Source: CAD feature listing. Evaluate the final solid. Frame: model axes, mm. A direction names the side the tool comes from. Round coordinates to 2 decimals unless told otherwise and drop trailing zeros. Loops run counter-clockwise (first coordinate to the right, second up) from the corner with the lowest first, then second, coordinate; pieces in that order, holes last. Notation, with made-up numbers: (69, 8) -> (108, 8) arc R11 cw to (108, 26) -> close; hole circle Ø11 at (60, -20). An arc over 180 degrees is marked (long way). Write item = value, one per line.
Autodesk Inventor part; units mm, degrees
ref_plane "YZ Plane" through (0, 0, 0) normal (1, 0, 0) x (0, 1, 0)
ref_plane "XZ Plane" through (0, 0, 0) normal (0, 1, 0) x (-1, 0, 0)
ref_plane "XY Plane" through (0, 0, 0) normal (0, 0, 1) x (1, 0, 0)
sketch "Base" plane through (0, 0, 0) normal (0, 0, 1) x (1, 0, 0)
  circle A0 centre (0, 0) radius 2
  line L0 (-4.5, 5) -> (4.5, 5)
  line L1 (4.5, 5) -> (4.5, -5)
  line L2 (4.5, -5) -> (-4.5, -5)
  line L3 (-4.5, -5) -> (-4.5, 5)
  line L4 (4.5, 0) -> (-4.5, 0) construction
  line L5 (4.5, 10) -> (41.5, 10)
  line L6 (41.5, 10) -> (41.5, -10)
  line L7 (41.5, -10) -> (4.5, -10)
  line L8 (4.5, -10) -> (4.5, 10)
  dimension "d0" = 4
  dimension "d1" = 10
  dimension "d2" = 9
  dimension "d3" = 20
  dimension "d4" = 37
extrude "Extrusion1" add sketch "Base" along normal mid plane 8 contours L0 L1 L2 L3
extrude "Extrusion2" add sketch "Base" along normal mid plane 15 contours L8 L5 L6 L7 L1
fillet "Fillet1" radius 4 2 edges at (-4.5, -5, 0) (-4.5, 5, 0)
fillet "Fillet2" radius 1 2 edges at (4.5, 10, 0) (4.5, -10, 0)
sketch "Sketch2" plane through (0, 0, 7.5) normal (0, 0, 1) x (1, 0, 0)
  arc A0 (4.5, -9) -> (5.5, -10) centre (5.5, -9) ccw
  line L0 (5.5, -10) -> (41.5, -10)
  line L1 (41.5, -10) -> (41.5, 10)
  line L2 (41.5, 10) -> (5.5, 10)
  arc A1 (5.5, 10) -> (4.5, 9) centre (5.5, 9) ccw
  line L3 (4.5, 9) -> (4.5, -9)
  line L4 (32.7998, 10) -> (33.5, 9)
  line L5 (33.5, 9) -> (41.5, 9)
  line L6 (41.5, -10) -> (41.5, 10)
  line L7 (41.5, 10) -> (5.5, 10)
  point P0 (0, 0)
  dimension "d11" = 1
  dimension "d12" = 8
  dimension "d13" = 125
extrude "Extrusion3" cut sketch "Sketch2" against normal up to surface (15 mm away) contours L5 L4 L2 L1
fillet "Fillet3" radius 0.5 2 edges at (32.7998, 10, 0) (33.5, 9, 0)
sketch "Sketch3" plane through (41.5, -10, 7.5) normal (1, 0, 0) x (0, 0, -1)
  line L0 (15, 19) -> (0, 19) construction
  line L1 (7.5, 19) -> (7.5, 0) construction
  line L2 (0, 0) -> (15, 0) construction
  line L3 (1.625, 14.625) -> (13.375, 14.625) construction
  line L4 (13.375, 14.625) -> (13.375, 4.375)
  line L5 (13.375, 4.375) -> (1.625, 4.375) construction
  line L6 (1.625, 4.375) -> (1.625, 14.625)
  line L7 (0, 0) -> (0, 19) construction
  line L8 (0, 9.5) -> (15, 9.5) construction
  line L9 (15, 19) -> (15, 0) construction
  arc A0 (13.375, 14.625) -> (1.625, 14.625) centre (7.5, 10.3724) ccw
  arc A1 (1.625, 4.375) -> (13.375, 4.375) centre (7.5, 8.6276) ccw
  point P0 (7.5, 10)
  point P1 (7.5, 14.625)
  point P2 (1.625, 9.5)
  point P3 (7.5, 17.625)
  point P4 (7.5, 1.375)
  dimension "d17" = 11.75
  dimension "d18" = 3
  dimension "d21" = 16.25
extrude "Extrusion4" add sketch "Sketch3" along normal blind 56.5
sketch "Sketch4" plane through (98, -10, 7.5) normal (1, 0, 0) x (0, 0, -1)
  line L0 (13.375, 4.375) -> (13.375, 14.625)
  arc A0 (13.375, 14.625) -> (1.625, 14.625) centre (7.5, 10.3724) ccw
  line L1 (1.625, 14.625) -> (1.625, 4.375)
  arc A1 (1.625, 4.375) -> (13.375, 4.375) centre (7.5, 8.6276) ccw
  arc A2 (12.875, 14.4598) -> (2.125, 14.4598) centre (7.5, 10.3724) ccw
  line L2 (12.875, 14.4598) -> (12.875, 4.5402)
  arc A3 (2.125, 4.5402) -> (12.875, 4.5402) centre (7.5, 8.6276) ccw
  line L3 (2.125, 4.5402) -> (2.125, 14.4598)
  point P0 (7.5, 10)
  dimension "d22" = 0.5
extrude "Extrusion5" add sketch "Sketch4" along normal blind 0.25 contours L2 A3 L3 A2
sketch "Sketch5" plane through (98.25, -10, 7.5) normal (1, 0, 0) x (0, 0, -1)
  arc A0 (13.375, 14.625) -> (1.625, 14.625) centre (7.5, 10.3724) ccw
  line L0 (1.625, 14.625) -> (1.625, 4.375)
  arc A1 (1.625, 4.375) -> (13.375, 4.375) centre (7.5, 8.6276) ccw
  line L1 (13.375, 4.375) -> (13.375, 14.625)
  point P0 (7.5, 10)
extrude "Extrusion6" add sketch "Sketch5" along normal blind 1.75
sketch "Sketch6" plane through (100, -10, 7.5) normal (1, 0, 0) x (0, 0, -1)
  circle A0 centre (7.5, 10) radius 4.5
  dimension "d27" = 9
extrude "Extrusion7" cut sketch "Sketch6" against normal blind 50
sketch "Sketch7" plane through (41.5, -5.625, 5.875) normal (0, 0, 1) x (1, 0, 0)
  line L0 (58.5, 0) -> (58.5, 10.25)
  line L1 (58.5, 5.125) -> (54.5, 5.125) construction
  circle A0 centre (52.5, 5.125) radius 2
  line L2 (52.5, 5.125) -> (54.5, 5.125) construction
  point P0 (-41.5, 5.625)
  dimension "d31" = 4
  dimension "d30" = 4
extrude "Extrusion8" cut sketch "Sketch7" against normal through all
properties part number "LA-T8-1215-50 105-64 Body"
1. Section query B-B (x = 78). Return the cut outline in (y, z) (3 decimals), then the cut area to 3 significant figures.
Evaluation:
outline = (-5.625, -5.875) -> (4.625, -5.875) arc R7.253 ccw to (4.625, 5.875) -> (-5.625, 5.875) arc R7.253 ccw to start; hole circle Ø9 at (0, 0)
area = 106 mm²
2. Set-up query: faces 1 (the face through (2, 1, -4)), 2 (the face through (2, -5, 0)), 3 (the face through (69.354, -8.624, -0.096)). Return all of +Z, -Z, +X, -X, +Y, -Y with unobstructed straight access to the full face (end or side cutting, diameter ignored); none if empty.
Evaluation:
face_1 = -Z, -X, +Y, -Y
face_2 = +Z, -Z, -X, -Y
face_3 = +X, -Y
3. Section query C-C (x = 94). Return the cut outline in (y, z) (3 decimals).
Evaluation:
outline = (-5.625, -5.875) -> (-2.5, -5.875) -> (-2.5, -3.742) arc R4.5 cw to (-2.5, 3.742) -> (-2.5, 5.875) -> (-5.625, 5.875) arc R7.253 ccw to start; (1.5, -5.875) -> (4.625, -5.875) arc R7.253 ccw to (4.625, 5.875) -> (1.5, 5.875) -> (1.5, 4.243) arc R4.5 cw to (1.5, -4.243) -> close
4. Mould query, pull axis X, two halves, no side actions, for faces 4 (the face through (94.923, -2.274, 5.06)), 5 (the face through (50, 0, 0)), 6 (the face through (2, 1, 4)). Classes: released by +X, released by -X, zero draft, split by the parting line, or undercut.
Evaluation:
face_4 = undercut
face_5 = released by +X
face_6 = zero draft
5. Line query: probe 1 along X at (y, z) = (-0.5, 5.25); probe 2 along Y at (x, z) = (0, 0.75); probe 3 along Z at (x, y) = (90.5, 1.5) (3 decimals). Output: solid intervals per line, ascending. Write a range as from..to.
Evaluation:
probe_1 = 4.5..92, 96..100
probe_2 = -5..-2, 2..5
probe_3 = -5.875..-4.243, 4.243..5.875
6. Section query D-D (x = 49). Return the cut outline in (y, z) (3 decimals), then the cut area to 3 significant figures.
Evaluation:
outline = (-5.625, -5.875) -> (4.625, -5.875) arc R7.253 ccw to (4.625, 5.875) -> (-5.625, 5.875) arc R7.253 ccw to start
area = 170 mm²
7. Contact query for flat-ended pins moving along their axis: pin 1 Ø3 at (x, y) = (65, -0.5) entering from -Z (3 decimals); pin 2 Ø1.5 at (y, z) = (-3.5, 1) entering from +X; pin 3 Ø1.5 at (x, z) = (1, 1.5) entering from -Y; pin 4 Ø2.5 at (x, y) = (0, 0) entering from +Z. Output: stop coordinate, or through.
Evaluation:
pin_1 = -5.875
pin_2 = 50
pin_3 = -5
pin_4 = through
